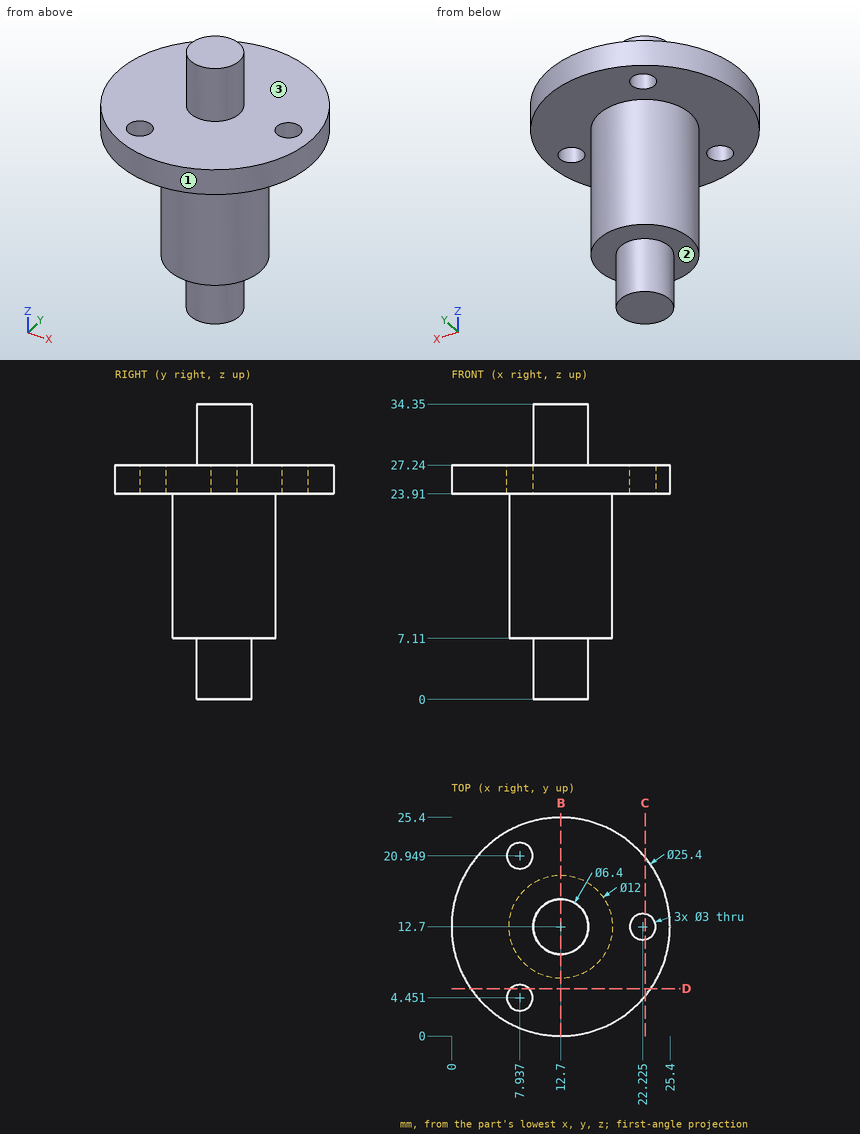
Input: dimensioned drawing with shaded views. Units: mm. Origin: part minimum x, y, z. A direction names the side the tool comes from. Coordinates: 2 decimals unless noted, no trailing zeros. Loops run counter-clockwise (first coordinate to the right, second up) from the corner with the lowest first, then second, coordinate; pieces in that order, holes last. Notation, with made-up numbers: (0.25, 8) -> (4.25, 8) arc R23 cw to (4.25, 31) -> close; hole circle Ø1 at (62.5, 88). An arc over 180 degrees is marked (long way). One line per item, written item: value. Start each with the question number.
Q1. Set-up query: the marked faces 1, 2 and 3. Return all of +Z, -Z, +X, -X, +Y, -Y with unobstructed straight access to the full face (end or side cutting, diameter ignored); none if empty.
Q2. Section query D-D, the plane y = 5.5. Return the cut outline in (x, z) (1 decimal).
Q3. Line query: line 1 along Z through (x, y) = (5.5, 16.25); line 2 along Z through (x, y) = (9.5, 12.25); line 3 along Y through (x, z) = (9.5, 27). Output: solid intervals per line, ascending.
Q4. Section query C-C, the plane x = 22.5. Return the cut outline in (y, z) (1 decimal).
Q5. Contact query for flat-ended pins moving along their axis: P1, Ø4, axis at y = 19, z = 24, coming from the +X side; P2, Ø2, axis at x = 12.5, z = 9.5, coming from the -Y side; P3, Ø1, axis at x = 17.5, z = 25.5, coming from the +Y side. Output: stop coordinate, or through.
Q6. Section query B-B, the plane x = 12.7. Return the cut outline in (y, z), and give its area (3 significant figures).
Results:
1. face 1: +Z, -Z
1. face 2: -Z
1. face 3: +Z
2. outline: (2.2, 23.9) -> (6.9, 23.9) -> (6.9, 27.2) -> (2.2, 27.2) -> close; (9, 23.9) -> (23.2, 23.9) -> (23.2, 27.2) -> (9, 27.2) -> close
3. line 1: 23.91 to 27.24
3. line 2: 7.11 to 27.24
3. line 3: 0.41 to 24.99
4. outline: (4.6, 23.9) -> (11.2, 23.9) -> (11.2, 27.2) -> (4.6, 27.2) -> close; (14.2, 23.9) -> (20.8, 23.9) -> (20.8, 27.2) -> (14.2, 27.2) -> close
5. P1: x = 24.65
5. P2: y = 6.7
5. P3: y = 24.65
6. outline: (0, 23.91) -> (6.7, 23.91) -> (6.7, 7.11) -> (9.5, 7.11) -> (9.5, 0) -> (15.9, 0) -> (15.9, 7.11) -> (18.7, 7.11) -> (18.7, 23.91) -> (25.4, 23.91) -> (25.4, 27.24) -> (15.9, 27.24) -> (15.9, 34.35) -> (9.5, 34.35) -> (9.5, 27.24) -> (0, 27.24) -> close
6. area: 377 mm^2
